Input: part model. Units: mm. Frame: model coordinates. A direction names the side the tool comes from. Give positions to 0.01 mm unless a question says otherwise; leave off trailing zeros. Write each loop counter-clockwise with the first axis right and the second up, starting at its lowest first coordinate (ties: lowest second). Pieces come first, ordered by that corner, then holes. Notation, with made-up numbers: (-28, 12.25) - (23, 12.25) arc R14 cw to (23, 28.25) - close; hole circle Ø5 at (64.5, 29.5). An arc over 180 degrees is marked (long way). Answer as CSV lines item,"result". Start each with the question number.
from build123d import *

# Parameters (mm, degrees)
F0_R     = 18.415
F1_DEPTH = 165.1
F2_R     = 5.08
F3_D     = 8.8
F4_R     = 4.4
F5_DEPTH = 6


with BuildPart() as f1:
    # F0 (on Top) → F1 (new body)
    with BuildSketch(Plane.XY):
        Circle(F0_R)
    extrude(amount=F1_DEPTH)

    # F2
    f2_edges = [f1.edges().sort_by_distance(p)[0] for p in [
        (-18.415, 0, 165.1),
        (-18.415, 0, 0),
    ]]
    fillet(f2_edges, radius=F2_R)

    # F3 (through all)
    with Locations(Plane(origin=(0, 0, 0), x_dir=(1, 0, 0), z_dir=(0, 0, -1))):
        with Locations((0, 0)):
            Hole(F3_D / 2)

    # F4 (on face) → F5 (cut)
    with BuildSketch(Plane.XY.offset(165.1)):
        Polygon((0.8534678569, 8.3279604917), (-6.7854914191, 4.9031050912), (-7.6389592759, -3.4248554005), (-0.8534678569, -8.3279604917), (6.7854914191, -4.9031050912), (7.6389592759, 3.4248554005), align=None)
        Circle(F4_R, mode=Mode.SUBTRACT)
    extrude(amount=-F5_DEPTH, mode=Mode.SUBTRACT)


solid = f1.part
1) Cut plane B-B on z = 22. Output: boundary loops of the cut face in (x, y) (3 decimals).
2) Reachability of faces 4 (the cylindrical face through (-4.197, -1.322, 80.664)), 5 (the flat face through (-7.206, 0.797, 162.142)) from +Z, -Z, +X, -X, +Y, -Y: full face, straight path, thin tool, end or side. Return the list, or none.
3) Cut plane A-A on y = 0. Output: boundary loops of the cut face in (x, z) (3 decimals), and give its area (3 significant figures).
4) Material intervals for line 1 (Y direction, x = 0, z = 64) (3 decimals); line 2 (X direction, y = -3, z = 107); line 3 (X direction, y = -1, z = 53), sorted ascending. Write a range as from..to.
5) Pull-direction query (Y, two-part tool) for faces 1 (the flat face through (6, 0, 0)), 2 (the flat face through (-4.294, -5.842, 162.142)), 3 (the cylindrical face through (-14.61, -11.21, 81.47)); classes: +Y half, -Y half, draft (parallel to the pull), parting line (faces both ways), or undercut.
6) Contact query for flat-ended pins moving along their axis: P1, Ø2, axis at x = 3.5, z = 35.5, coming from the -Y side; P2, Ø10, axis at y = 10.5, z = 92.5, coming from the -X side; P3, Ø8, axis at y = -7.5, z = 28.5, coming from the +X side; P4, Ø8, axis at x = 0, y = 0, coming from the -Z side. Output: stop coordinate, or through.
Numbers:
1,outline,"circle Ø36.83 at (0, 0); hole circle Ø8.8 at (0, 0)"
2,face 4,"+Z, -Z"
2,face 5,"+Z"
3,outline,"(-18.415, 5.08) arc R5.08 ccw to (-13.335, 0) - (-4.4, 0) - (-4.4, 159.1) - (-7.288, 159.1) - (-7.288, 165.1) - (-13.335, 165.1) arc R5.08 ccw to (-18.415, 160.02) - close; (4.4, 0) - (13.335, 0) arc R5.08 ccw to (18.415, 5.08) - (18.415, 160.02) arc R5.08 ccw to (13.335, 165.1) - (7.288, 165.1) - (7.288, 159.1) - (4.4, 159.1) - close"
3,area,"4,570 mm²"
4,line 1,"y = -18.415..-4.4, 4.4..18.415"
4,line 2,"x = -18.17..-3.22, 3.22..18.17"
4,line 3,"x = -18.39..-4.28, 4.28..18.39"
5,face 1,"draft"
5,face 2,"undercut"
5,face 3,"parting line"
6,P1,"stops at y = -18.24"
6,P2,"stops at x = -17.57"
6,P3,"stops at x = 18.08"
6,P4,"passes through"
